For this review, take the finished solid that the model builds, in its own axes (mm). A direction names the side the tool comes from. Round coordinates to 2 decimals unless told otherwise and drop trailing zeros. Order: outer loops, then holes, each group sorted by start corner. A loop starts at its lowest first (then second) coordinate and runs counter-clockwise, first axis right, second up. Notation, with made-up numbers: M 2.5,10.5 L 33.5,10.5 A13 cw 33.5,14.5 Z; hole C -22.5,61.25 d2. An arc over 180 degrees is marked long. Answer as a JSON object with one key per item and string values.
from build123d import *

# Parameters (mm, degrees)
SKETCH3_W           = 155
SKETCH3_H           = 77
BOSS_EXTRUDE1_DEPTH = 28
SKETCH5_W           = 143
SKETCH5_H           = 17
CUT_EXTRUDE1_DEPTH  = 113.77965242
BOSS_EXTRUDE3_REACH = 91.289
SKETCH12_R          = 18.25
SKETCH15_R          = 16.25
CUT_EXTRUDE4_DEPTH  = 27
CUT_EXTRUDE5_REACH  = 92.953
SKETCH16_R          = 3.5
SKETCH16_W          = 38
SKETCH16_H          = 53
SKETCH19_W          = 10
SKETCH19_H          = 12
CUT_EXTRUDE6_DEPTH  = 5
CUT_EXTRUDE7_DEPTH  = 163.145767752
CUT_EXTRUDE8_REACH  = 92.953
SKETCH23_R          = 1.625
SKETCH28_W          = 24
SKETCH28_H          = 18.5
BOSS_EXTRUDE4_DEPTH = 4
SKETCH29_W          = 20
SKETCH29_H          = 14.5
CUT_EXTRUDE11_DEPTH = 4
SKETCH30_R          = 3.25
CUT_EXTRUDE12_DEPTH = 1.5
CUT_EXTRUDE13_REACH = 164.146
SKETCH31_R          = 1.55
CUT_EXTRUDE14_REACH = 164.146
SKETCH32_R          = 1.55
SKETCH33_W          = 18
SKETCH33_H          = 6
CUT_EXTRUDE15_DEPTH = 3
SKETCH34_W          = 18
SKETCH34_H          = 6
CUT_EXTRUDE16_DEPTH = 3
SKETCH35_R          = 3.75
CUT_EXTRUDE17_DEPTH = 90.288857088
CUT_EXTRUDE18_REACH = 92.953
SKETCH36_R          = 1.75


with BuildPart() as part:
    # Sketch3 → Boss-Extrude1 (new body)
    with BuildSketch(Plane(origin=(0, 0, 0), x_dir=(1, 0, 0), z_dir=(0, 1, 0))):
        Rectangle(SKETCH3_W, SKETCH3_H)
    extrude(amount=BOSS_EXTRUDE1_DEPTH)

    # Sketch5 → Cut-Extrude1 (cut, through all)
    with BuildSketch(Plane.XY.offset(38.5)):
        with Locations((0, 14.5)):
            Rectangle(SKETCH5_W, SKETCH5_H)
    extrude(amount=-CUT_EXTRUDE1_DEPTH, mode=Mode.SUBTRACT)

    # Sketch12 → Boss-Extrude3 (add, up to next)
    with BuildSketch(Plane(origin=(0, 6, 0), x_dir=(1, 0, 0), z_dir=(0, 1, 0)), mode=Mode.PRIVATE) as boss_extrude3_sk1:
        with Locations(Location((0, 0, 0), (0, 0, 90))):
            Circle(SKETCH12_R)
    boss_extrude3_tool1 = extrude(boss_extrude3_sk1.sketch, amount=BOSS_EXTRUDE3_REACH, mode=Mode.PRIVATE) - part.part
    add(boss_extrude3_tool1.solids().sort_by_distance((0, 6, 0))[0])

    # Sketch15 → Cut-Extrude4 (cut)
    with BuildSketch(Plane(origin=(0, 28, 0), x_dir=(1, 0, 0), z_dir=(0, 1, 0))):
        with Locations(Location((0, 0, 0), (0, 0, 270))):
            Circle(SKETCH15_R)
    extrude(amount=-CUT_EXTRUDE4_DEPTH, mode=Mode.SUBTRACT)

    # Sketch16 → Cut-Extrude5 (cut, up to next)
    with BuildSketch(Plane(origin=(0, 28, 0), x_dir=(1, 0, 0), z_dir=(0, 1, 0)), mode=Mode.PRIVATE) as cut_extrude5_sk1:
        with Locations(Location((-12.5, 26.5, 0), (0, 0, 270))):
            Circle(SKETCH16_R)
    cut_extrude5_tool1 = extrude(cut_extrude5_sk1.sketch, amount=-CUT_EXTRUDE5_REACH, mode=Mode.PRIVATE) & part.part
    # Sketch16 → Cut-Extrude5 (cut, up to next)
    with BuildSketch(Plane(origin=(0, 28, 0), x_dir=(1, 0, 0), z_dir=(0, 1, 0)), mode=Mode.PRIVATE) as cut_extrude5_sk2:
        with Locations(Location((12.5, 26.5, 0), (0, 0, 270))):
            Circle(SKETCH16_R)
    cut_extrude5_tool2 = extrude(cut_extrude5_sk2.sketch, amount=-CUT_EXTRUDE5_REACH, mode=Mode.PRIVATE) & part.part
    # Sketch16 → Cut-Extrude5 (cut, up to next)
    with BuildSketch(Plane(origin=(0, 28, 0), x_dir=(1, 0, 0), z_dir=(0, 1, 0)), mode=Mode.PRIVATE) as cut_extrude5_sk3:
        with Locations(Location((12.5, -26.5, 0), (0, 0, 270))):
            Circle(SKETCH16_R)
    cut_extrude5_tool3 = extrude(cut_extrude5_sk3.sketch, amount=-CUT_EXTRUDE5_REACH, mode=Mode.PRIVATE) & part.part
    # Sketch16 → Cut-Extrude5 (cut, up to next)
    with BuildSketch(Plane(origin=(0, 28, 0), x_dir=(1, 0, 0), z_dir=(0, 1, 0)), mode=Mode.PRIVATE) as cut_extrude5_sk4:
        with Locations(Location((-12.5, -26.5, 0), (0, 0, 270))):
            Circle(SKETCH16_R)
    cut_extrude5_tool4 = extrude(cut_extrude5_sk4.sketch, amount=-CUT_EXTRUDE5_REACH, mode=Mode.PRIVATE) & part.part
    # Sketch16 → Cut-Extrude5 (cut, up to next)
    with BuildSketch(Plane(origin=(0, 28, 0), x_dir=(1, 0, 0), z_dir=(0, 1, 0)), mode=Mode.PRIVATE) as cut_extrude5_sk5:
        with Locations((-42.5, 0)):
            Rectangle(SKETCH16_W, SKETCH16_H)
    cut_extrude5_tool5 = extrude(cut_extrude5_sk5.sketch, amount=-CUT_EXTRUDE5_REACH, mode=Mode.PRIVATE) & part.part
    # Sketch16 → Cut-Extrude5 (cut, up to next)
    with BuildSketch(Plane(origin=(0, 28, 0), x_dir=(1, 0, 0), z_dir=(0, 1, 0)), mode=Mode.PRIVATE) as cut_extrude5_sk6:
        with Locations((42.5, 0)):
            Rectangle(SKETCH16_W, SKETCH16_H)
    cut_extrude5_tool6 = extrude(cut_extrude5_sk6.sketch, amount=-CUT_EXTRUDE5_REACH, mode=Mode.PRIVATE) & part.part
    add(cut_extrude5_tool1.solids().sort_by_distance((-12.5, 28, -26.5))[0], mode=Mode.SUBTRACT)
    add(cut_extrude5_tool2.solids().sort_by_distance((12.5, 28, -26.5))[0], mode=Mode.SUBTRACT)
    add(cut_extrude5_tool3.solids().sort_by_distance((12.5, 28, 26.5))[0], mode=Mode.SUBTRACT)
    add(cut_extrude5_tool4.solids().sort_by_distance((-12.5, 28, 26.5))[0], mode=Mode.SUBTRACT)
    add(cut_extrude5_tool5.solids().sort_by_distance((-42.5, 28, 0))[0], mode=Mode.SUBTRACT)
    add(cut_extrude5_tool6.solids().sort_by_distance((42.5, 28, 0))[0], mode=Mode.SUBTRACT)

    # Sketch19 → Cut-Extrude6 (cut)
    with BuildSketch(Plane.XZ):
        with Locations((-72.5, 0)):
            Rectangle(SKETCH19_W, SKETCH19_H)
        with Locations((72.5, 0)):
            Rectangle(SKETCH19_W, SKETCH19_H)
    extrude(amount=-CUT_EXTRUDE6_DEPTH, mode=Mode.SUBTRACT)

    # Sketch22 → Cut-Extrude7 (cut, through all)
    with BuildSketch(Plane.ZY.offset(77.5)):
        Polygon((-38.5, 0), (-38.5, 12), (-27.5, 0), align=None)
        Polygon((38.5, 12), (27.5, 0), (38.5, 0), align=None)
    extrude(amount=-CUT_EXTRUDE7_DEPTH, mode=Mode.SUBTRACT)

    # Sketch23 → Cut-Extrude8 (cut, up to next)
    with BuildSketch(Plane.XZ, mode=Mode.PRIVATE) as cut_extrude8_sk1:
        with Locations(Location((39.25, 0, 0), (0, 0, 270))):
            Circle(SKETCH23_R)
    cut_extrude8_tool1 = extrude(cut_extrude8_sk1.sketch, amount=-CUT_EXTRUDE8_REACH, mode=Mode.PRIVATE) & part.part
    # Sketch23 → Cut-Extrude8 (cut, up to next)
    with BuildSketch(Plane.XZ, mode=Mode.PRIVATE) as cut_extrude8_sk2:
        with Locations(Location((-39.25, 0, 0), (0, 0, 270))):
            Circle(SKETCH23_R)
    cut_extrude8_tool2 = extrude(cut_extrude8_sk2.sketch, amount=-CUT_EXTRUDE8_REACH, mode=Mode.PRIVATE) & part.part
    add(cut_extrude8_tool1.solids().sort_by_distance((39.25, 0, 0))[0], mode=Mode.SUBTRACT)
    add(cut_extrude8_tool2.solids().sort_by_distance((-39.25, 0, 0))[0], mode=Mode.SUBTRACT)

    # Sketch28 → Boss-Extrude4 (add)
    with BuildSketch(Plane(origin=(0, 6, 0), x_dir=(1, 0, 0), z_dir=(0, 1, 0))):
        with Locations((-39.25, 0)):
            Rectangle(SKETCH28_W, SKETCH28_H)
    extrude(amount=BOSS_EXTRUDE4_DEPTH)

    # Sketch29 → Cut-Extrude11 (cut)
    with BuildSketch(Plane(origin=(0, 10, 0), x_dir=(1, 0, 0), z_dir=(0, 1, 0))):
        with Locations((-39.25, 0)):
            Rectangle(SKETCH29_W, SKETCH29_H)
    extrude(amount=-CUT_EXTRUDE11_DEPTH, mode=Mode.SUBTRACT)

    # Sketch30 → Cut-Extrude12 (cut)
    with BuildSketch(Plane(origin=(0, 6, 0), x_dir=(1, 0, 0), z_dir=(0, 1, 0))):
        with Locations(Location((-39.25, 0, 0), (0, 0, 270))):
            Circle(SKETCH30_R)
    extrude(amount=-CUT_EXTRUDE12_DEPTH, mode=Mode.SUBTRACT)

    # Sketch31 → Cut-Extrude13 (cut, up to next)
    with BuildSketch(Plane(origin=(77.5, 0, 0), x_dir=(0, 0, -1), z_dir=(1, 0, 0)), mode=Mode.PRIVATE) as cut_extrude13_sk1:
        with Locations((-8.55, 16)):
            Circle(SKETCH31_R)
    cut_extrude13_tool1 = extrude(cut_extrude13_sk1.sketch, amount=-CUT_EXTRUDE13_REACH, mode=Mode.PRIVATE) & part.part
    # Sketch31 → Cut-Extrude13 (cut, up to next)
    with BuildSketch(Plane(origin=(77.5, 0, 0), x_dir=(0, 0, -1), z_dir=(1, 0, 0)), mode=Mode.PRIVATE) as cut_extrude13_sk2:
        with Locations((8.55, 16)):
            Circle(SKETCH31_R)
    cut_extrude13_tool2 = extrude(cut_extrude13_sk2.sketch, amount=-CUT_EXTRUDE13_REACH, mode=Mode.PRIVATE) & part.part
    add(cut_extrude13_tool1.solids().sort_by_distance((77.5, 16, 8.55))[0], mode=Mode.SUBTRACT)
    add(cut_extrude13_tool2.solids().sort_by_distance((77.5, 16, -8.55))[0], mode=Mode.SUBTRACT)

    # Sketch32 → Cut-Extrude14 (cut, up to next)
    with BuildSketch(Plane.ZY.offset(77.5), mode=Mode.PRIVATE) as cut_extrude14_sk1:
        with Locations(Location((-8.55, 16, 0), (0, 0, 180))):
            Circle(SKETCH32_R)
    cut_extrude14_tool1 = extrude(cut_extrude14_sk1.sketch, amount=-CUT_EXTRUDE14_REACH, mode=Mode.PRIVATE) & part.part
    # Sketch32 → Cut-Extrude14 (cut, up to next)
    with BuildSketch(Plane.ZY.offset(77.5), mode=Mode.PRIVATE) as cut_extrude14_sk2:
        with Locations(Location((8.55, 16, 0), (0, 0, 180))):
            Circle(SKETCH32_R)
    cut_extrude14_tool2 = extrude(cut_extrude14_sk2.sketch, amount=-CUT_EXTRUDE14_REACH, mode=Mode.PRIVATE) & part.part
    add(cut_extrude14_tool1.solids().sort_by_distance((-77.5, 16, -8.55))[0], mode=Mode.SUBTRACT)
    add(cut_extrude14_tool2.solids().sort_by_distance((-77.5, 16, 8.55))[0], mode=Mode.SUBTRACT)

    # Sketch33 → Cut-Extrude15 (cut)
    with BuildSketch(Plane.ZY.offset(77.5)):
        with Locations((0, 25)):
            Rectangle(SKETCH33_W, SKETCH33_H)
    extrude(amount=-CUT_EXTRUDE15_DEPTH, mode=Mode.SUBTRACT)

    # Sketch34 → Cut-Extrude16 (cut)
    with BuildSketch(Plane(origin=(77.5, 0, 0), x_dir=(0, 0, -1), z_dir=(1, 0, 0))):
        with Locations((0, 25)):
            Rectangle(SKETCH34_W, SKETCH34_H)
    extrude(amount=-CUT_EXTRUDE16_DEPTH, mode=Mode.SUBTRACT)

    # Sketch35 → Cut-Extrude17 (cut, through all)
    with BuildSketch(Plane(origin=(0, 6, 0), x_dir=(1, 0, 0), z_dir=(0, 1, 0))):
        with Locations(Location((62.75, 0, 0), (0, 0, 270))):
            Circle(SKETCH35_R)
    extrude(amount=-CUT_EXTRUDE17_DEPTH, mode=Mode.SUBTRACT)

    # Sketch36 → Cut-Extrude18 (cut, up to next)
    with BuildSketch(Plane(origin=(0, 28, 0), x_dir=(1, 0, 0), z_dir=(0, 1, 0)), mode=Mode.PRIVATE) as cut_extrude18_sk1:
        with Locations(Location((-63.5, -34.5, 0), (0, 0, 270))):
            Circle(SKETCH36_R)
    cut_extrude18_tool1 = extrude(cut_extrude18_sk1.sketch, amount=-CUT_EXTRUDE18_REACH, mode=Mode.PRIVATE) & part.part
    # Sketch36 → Cut-Extrude18 (cut, up to next)
    with BuildSketch(Plane(origin=(0, 28, 0), x_dir=(1, 0, 0), z_dir=(0, 1, 0)), mode=Mode.PRIVATE) as cut_extrude18_sk2:
        with Locations(Location((-68.5, 18, 0), (0, 0, 270))):
            Circle(SKETCH36_R)
    cut_extrude18_tool2 = extrude(cut_extrude18_sk2.sketch, amount=-CUT_EXTRUDE18_REACH, mode=Mode.PRIVATE) & part.part
    # Sketch36 → Cut-Extrude18 (cut, up to next)
    with BuildSketch(Plane(origin=(0, 28, 0), x_dir=(1, 0, 0), z_dir=(0, 1, 0)), mode=Mode.PRIVATE) as cut_extrude18_sk3:
        with Locations(Location((-35.5, -34.5, 0), (0, 0, 270))):
            Circle(SKETCH36_R)
    cut_extrude18_tool3 = extrude(cut_extrude18_sk3.sketch, amount=-CUT_EXTRUDE18_REACH, mode=Mode.PRIVATE) & part.part
    # Sketch36 → Cut-Extrude18 (cut, up to next)
    with BuildSketch(Plane(origin=(0, 28, 0), x_dir=(1, 0, 0), z_dir=(0, 1, 0)), mode=Mode.PRIVATE) as cut_extrude18_sk4:
        with Locations(Location((65.5, -18.75, 0), (0, 0, 270))):
            Circle(SKETCH36_R)
    cut_extrude18_tool4 = extrude(cut_extrude18_sk4.sketch, amount=-CUT_EXTRUDE18_REACH, mode=Mode.PRIVATE) & part.part
    # Sketch36 → Cut-Extrude18 (cut, up to next)
    with BuildSketch(Plane(origin=(0, 28, 0), x_dir=(1, 0, 0), z_dir=(0, 1, 0)), mode=Mode.PRIVATE) as cut_extrude18_sk5:
        with Locations(Location((65.5, 18.75, 0), (0, 0, 270))):
            Circle(SKETCH36_R)
    cut_extrude18_tool5 = extrude(cut_extrude18_sk5.sketch, amount=-CUT_EXTRUDE18_REACH, mode=Mode.PRIVATE) & part.part
    add(cut_extrude18_tool1.solids().sort_by_distance((-63.5, 28, 34.5))[0], mode=Mode.SUBTRACT)
    add(cut_extrude18_tool2.solids().sort_by_distance((-68.5, 28, -18))[0], mode=Mode.SUBTRACT)
    add(cut_extrude18_tool3.solids().sort_by_distance((-35.5, 28, 34.5))[0], mode=Mode.SUBTRACT)
    add(cut_extrude18_tool4.solids().sort_by_distance((65.5, 28, 18.75))[0], mode=Mode.SUBTRACT)
    add(cut_extrude18_tool5.solids().sort_by_distance((65.5, 28, -18.75))[0], mode=Mode.SUBTRACT)


solid = part.part
1) Mouldability with a two-part tool opening along X and no side actions: class faces 1 (the cylindrical face through (63.79, 25.54, 18.37)), 2 (the flat face through (-1, 0, 0)), 3 (the flat face through (42, 26, -26.5)), 4 (the flat face through (-77.5, 14, 1)) as +X half, -X half, draft (parallel to the pull), parting line (faces both ways), or undercut.
Geometry check:
{"face 1": "undercut", "face 2": "draft", "face 3": "undercut", "face 4": "-X half"}
2) Add section C-C on y = 24.5. State how many separate pieces and enclosed holes the cut face has, and give its area (3 significant figures).
Geometry check:
{"separate pieces": "1", "enclosed holes": "12", "area": "6,770 mm²"}
3) For L1, parallel to X at y = 18.5, z = 1; L2, parallel to X at y = 5.7, z = 0 (3 decimals); L3, parallel to X at y = 26.5, z = 18.5, list the stretches that pass through material, from the lowest coordinate up.
Geometry check:
{"L1": "x = -77.5 to -71.5, -18.22 to -16.22, 16.22 to 18.22, 71.5 to 77.5", "L2": "x = -77.5 to -42.5, -36 to -16.25, 16.25 to 37.625, 40.875 to 59, 66.5 to 77.5", "L3": "x = -77.5 to -61.5, -23.5 to 23.5, 61.5 to 63.77, 67.23 to 77.5"}
4) Add section B-B on x = 32. State the section outline as (y, z) points, and give its area (3 significant figures).
Geometry check:
{"outline": "M 0,-27.5 L 6,-33 L 6,33 L 0,27.5 Z; M 23,-38.5 L 28,-38.5 L 28,-26.5 L 23,-26.5 Z; M 23,26.5 L 28,26.5 L 28,38.5 L 23,38.5 Z", "area": "483 mm²"}
5) Insertion check: P1, Ø5, axis at x = 53.5, z = 23.5, coming from the +Y side; P2, Ø4, axis at y = 2.5, z = 1.5, coming from the +X side; P3, Ø3, axis at y = 16, z = 8.55, coming from the -X side. Each pin has a flat end and moves straight along its axis. Give the tip position at first contact, or say it passes through.
Geometry check:
{"P1": "stops at y = 6", "P2": "stops at x = 67.5", "P3": "stops at x = -16.83"}
6) Add section A-A on y = 16. State the section outline as (x, z) points, and give its area (3 significant figures).
Geometry check:
{"outline": "M -77.5,-38.5 L -71.5,-38.5 L -71.5,-10.1 L -77.5,-10.1 Z; M -77.5,-7 L -71.5,-7 L -71.5,7 L -77.5,7 Z; M -77.5,10.1 L -71.5,10.1 L -71.5,38.5 L -77.5,38.5 Z; C 0,0 d36.5; M 71.5,-38.5 L 77.5,-38.5 L 77.5,-10.1 L 71.5,-10.1 Z; M 71.5,-7 L 77.5,-7 L 77.5,7 L 71.5,7 Z; M 71.5,10.1 L 77.5,10.1 L 77.5,38.5 L 71.5,38.5 Z; hole C 0,0 d32.5", "area": "1,070 mm²"}
7) Machinability: for faces 5 (the flat face through (-17, 23, -8)), 6 (the flat face through (-73, 2, -6)), 7 (the flat face through (72, 2, 6)), 8 (the flat face through (-39, 8, 7.25)), 9 (the flat face through (-74.5, 25, 0)), which of the approach directions +Z, -Z, +X, -X, +Y, -Y give a long, thin tool a straight path to every point of the face, cutting with its end or side? Answer none if there is none.
Geometry check:
{"face 5": "none", "face 6": "-X, -Y", "face 7": "+X, -Y", "face 8": "+Y", "face 9": "-X, +Y"}
